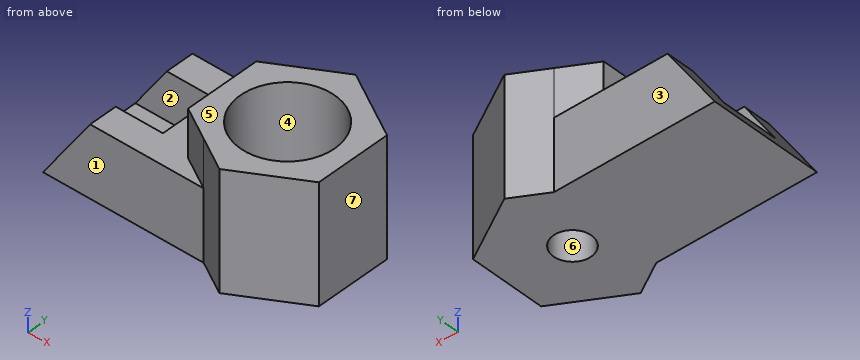
from build123d import *

# Parameters (mm, degrees)
F1_DEPTH  = 30
F2_DEPTH  = 50
F3_R      = 20
F4_DEPTH  = 36
F5_R      = 8
F6_DEPTH  = 14.001
F7_W      = 40
F7_H      = 24
F8_DEPTH  = 20
F10_DEPTH = 56.001


with BuildPart() as f1:
    # F0 (on Top) → F1 (new body)
    with BuildSketch(Plane.XY):
        Polygon((-27.712813, 16), (-13.856406, 24), (-82, 24), (-82, -24), (-13.856406, -24), (-27.712813, -16), align=None)
    extrude(amount=F1_DEPTH)

    # F0 (on Top) → F2 (join)
    with BuildSketch(Plane.XY):
        Polygon((27.712813, 16), (0, 32), (-13.856406, 24), (-27.712813, 16), (-27.712813, -16), (-13.856406, -24), (0, -32), (27.712813, -16), align=None)
    extrude(amount=F2_DEPTH)

    # F3 (on face) → F4 (cut)
    with BuildSketch(Plane.XY.offset(50)):
        Circle(F3_R)
    extrude(amount=-F4_DEPTH, mode=Mode.SUBTRACT)

    # F5 (on face) → F6 (cut, through all)
    with BuildSketch(Plane.XY.offset(14)):
        Circle(F5_R)
    extrude(amount=-F6_DEPTH, mode=Mode.SUBTRACT)

    # F7 (on face) → F8 (cut)
    with BuildSketch(Plane.XY.offset(30)):
        with Locations((-62, 0)):
            Rectangle(F7_W, F7_H)
    extrude(amount=-F8_DEPTH, mode=Mode.SUBTRACT)

    # F9 (on face) → F10 (cut, through all)
    with BuildSketch(Plane.XZ.offset(24)):
        Polygon((-82, 30), (-82, 0), (-62, 30), align=None)
    extrude(amount=-F10_DEPTH, mode=Mode.SUBTRACT)


solid = f1.part
Model file for the job. Use its own axes, mm. Face numbers are marked on the shaded views. A direction names the side the tool comes from. Round coordinates to 2 decimals unless told otherwise and drop trailing zeros. Loops run counter-clockwise (first coordinate to the right, second up) from the corner with the lowest first, then second, coordinate; pieces in that order, holes last.
1. Tool access for the marked faces 1, 2 and 3: list every direction of +Z, -Z, +X, -X, +Y, -Y with a clear straight run to the whole face (end or side of a thin tool).
Check values:
face 1: +Z, -Z, -X, -Y
face 2: +Z, -X
face 3: +Z, -Z, -X, +Y
2. Drop flat-ended pins along their axis: P1, Ø24, axis at x = 0, y = 0, coming from the +Z side; P2, Ø1, axis at y = -10, z = 33, coming from the -X side; P3, Ø6, axis at y = 5, z = 24.5, coming from the -X side. Give the stop position or say it passes through.
Check values:
P1: stops at z = 14
P2: stops at x = -27.71
P3: stops at x = -42
3. Band-saw the part on B-B, the plane y = 0. List the corners of the cut face in (x, z), and give its area (3 significant figures).
Check values:
outline: (-82, 0) - (-8, 0) - (-8, 14) - (-20, 14) - (-20, 50) - (-27.71, 50) - (-27.71, 30) - (-42, 30) - (-42, 10) - (-75.33, 10) - close; (8, 0) - (27.71, 0) - (27.71, 50) - (20, 50) - (20, 14) - (8, 14) - close
area: 1,900 mm2
4. Band-saw the part on C-C, the plane x = -73. List the corners of the cut face in (y, z).
Check values:
outline: (-24, 0) - (24, 0) - (24, 13.5) - (12, 13.5) - (12, 10) - (-12, 10) - (-12, 13.5) - (-24, 13.5) - close
5. Band-saw the part on D-D, the plane z = 7.5. List the corners of the cut face in (x, y).
Check values:
outline: (-77, -24) - (-13.86, -24) - (0, -32) - (27.71, -16) - (27.71, 16) - (0, 32) - (-13.86, 24) - (-77, 24) - close; hole circle Ø16 at (0, 0)
6. Wall check: probe 1 along Y at (x, z) = (-66.5, 16.5); probe 2 along Y at (x, z) = (0, 27); probe 3 along Z at (x, y) = (7, 17). Give the ranges that are in metal, low to high.
Check values:
probe 1: y = -24 to -12, 12 to 24
probe 2: y = -32 to -20, 20 to 32
probe 3: z = 0 to 14
7. Band-saw the part on A-A, the plane z = 31.5. List the corners of the cut face in (x, y).
Check values:
outline: (-27.71, -16) - (0, -32) - (27.71, -16) - (27.71, 16) - (0, 32) - (-27.71, 16) - close; hole circle Ø40 at (0, 0)
8. Mould opens along X. For the marked faces 4, 5, 6 and 7 say: +X half, -X half, draft (parallel to the pull), parting line (faces both ways), or undercut.
Check values:
face 4: undercut
face 5: draft
face 6: undercut
face 7: +X half
